Could you check a few things on this model? Use its own coordinates, in mm. A direction names the side the tool comes from. Round coordinates to 2 decimals unless told otherwise and drop trailing zeros. Write each loop counter-clockwise with the first axis right and the second up, starting at its lowest first coordinate (ties: lowest second). Pieces come first, ordered by that corner, then holes. Notation, with made-up numbers: (51, -3) -> (79, -3) arc R23 ccw to (79, 18) -> close; hole circle Ø2 at (73, -39.5). An arc over 180 degrees is marked (long way). Answer as CSV lines item,"result". Start each with the question number.
Q1. Imagine slicing it at A-A on y = 108. Please give me the cut outline in (x, z).
Q2. If we mould it in two halves opening along X, with no side actions, what happens to faces 6 (the cylindrical face through (54.55, 63.2, 0.93)), 7 (the cylindrical face through (-53.253, 56.857, 3.226)), 8 (the flat face through (-49.5, 73, 7)), 9 (the flat face through (-1, 115, 2))? For each: pulls with the +X half, pulls with the -X half, needs draft (parallel to the pull), parting line crosses it, or undercut.
Q3. Imagine slicing it at D-D on y = 62. Please give me the cut outline in (x, z), and give its area (3 significant figures).
Q4. Imagine slicing it at B-B on x = 0. Please give me the cut outline in (y, z).
Q5. Imagine slicing it at C-C on z = 6.25. Please give me the cut outline in (x, y), and give its area (3 significant figures).
Q6. Will these pins go through, and if not, where does the flat tip stop? pin 1 Ø4 at (x, y) = (59, 55.5) entering from -Z; pin 2 Ø10.5 at (x, y) = (0, 108) entering from +Z; pin 3 Ø2.5 at (x, z) = (-7, 3.5) entering from -Y; pin 4 Ø6 at (x, y) = (-50, 108) entering from +Z.
Q7. For faces 1 (the flat face through (-63.5, 81, 2)), 2 (the flat face through (-35.5, 73, 5)), 3 (the flat face through (59, 60, 1.5)), 4 (the flat face through (42, 74, 10)), 5 (the flat face through (-43, 100, 7)), which set-ups out of +Z, -Z, +X, -X, +Y, -Y let a thin tool reach every point of the face, with its end or its side?
Q8. If I drill on line 1 (X direction, y = 57, z = 0.45); line 2 (Y direction, x = 50, z = 2.5); line 3 (Y direction, x = 0, z = 1.9), over which ranges is the centre line in solid material (lowest first)? Write a range as [from, to].
from build123d import *

# Parameters (mm, degrees)
SKETCH2_R            = 3.25
BOSS_EXTRUDE2_DEPTH  = 5
SKETCH4_W            = 14
SKETCH4_H            = 53
RIBS_DEPTH           = 5
ANGLE_CUT_DEPTH      = 132.746916472
ANGLE_CUT_DEPTH_BACK = 132.746916472
SKETCH3_R            = 6.5
COUNTERBORE_DEPTH    = 1.5
SKETCH6_R            = 3.25
BOLT_THRU_HOLE_DEPTH = 105.895123001


with BuildPart() as part:
    # Sketch2 → Boss-Extrude2 (new body)
    with BuildSketch(Plane.XY):
        Polygon((-63.5, 47), (-63.5, 115), (63.5, 115), (63.5, 47), (35.5, 47), (35.5, 100), (-35.5, 100), (-35.5, 47), align=None)
        with Locations((-50, 108)):
            Circle(SKETCH2_R, mode=Mode.SUBTRACT)
        with Locations((50, 108)):
            Circle(SKETCH2_R, mode=Mode.SUBTRACT)
        with Locations((0, 108)):
            Circle(SKETCH2_R, mode=Mode.SUBTRACT)
    extrude(amount=BOSS_EXTRUDE2_DEPTH)

    # Sketch4 → Ribs (add)
    with BuildSketch(Plane.XY.offset(5)):
        with Locations((-42.5, 73.5)):
            Rectangle(SKETCH4_W, SKETCH4_H)
        with Locations((42.5, 73.5)):
            Rectangle(SKETCH4_W, SKETCH4_H)
    extrude(amount=RIBS_DEPTH)

    # Sketch5 → Angle Cut (cut, two sides: drawn at the far end of the back side and taken through both)
    with BuildSketch(Plane(origin=(0, 0, 0), x_dir=(0, 0, -1), z_dir=(1, 0, 0)).offset(-ANGLE_CUT_DEPTH_BACK)):
        Polygon((0, 47), (0, 65), (-0.628573851, 47), align=None)
    extrude(amount=ANGLE_CUT_DEPTH + ANGLE_CUT_DEPTH_BACK, mode=Mode.SUBTRACT)

    # Sketch3 → Counterbore (cut)
    with BuildSketch(Plane(origin=(0, 93.494633495, 0), x_dir=(-1, 0, 0), z_dir=(0, 0, 1))):
        with Locations(Location((56.5, 36.494633495, 0), (0, 0, 270))):
            Circle(SKETCH3_R)
        with Locations(Location((-56.5, 36.494633495, 0), (0, 0, 270))):
            Circle(SKETCH3_R)
    extrude(amount=COUNTERBORE_DEPTH, mode=Mode.SUBTRACT)

    # Sketch6 → Bolt thru-hole (cut, through all)
    with BuildSketch(Plane(origin=(0, 129.889907886, 0), x_dir=(-1, 0, 0), z_dir=(0, 0, 1))):
        with Locations((-56.5, 72.889907886)):
            Circle(SKETCH6_R)
        with Locations((56.5, 72.889907886)):
            Circle(SKETCH6_R)
    extrude(amount=BOLT_THRU_HOLE_DEPTH, mode=Mode.SUBTRACT)


solid = part.part
Checks:
1,outline,"(-63.5, 0) -> (-53.25, 0) -> (-53.25, 5) -> (-63.5, 5) -> close; (-46.75, 0) -> (-3.25, 0) -> (-3.25, 5) -> (-46.75, 5) -> close; (3.25, 0) -> (46.75, 0) -> (46.75, 5) -> (3.25, 5) -> close; (53.25, 0) -> (63.5, 0) -> (63.5, 5) -> (53.25, 5) -> close"
2,face 6,"undercut"
2,face 7,"undercut"
2,face 8,"pulls with the -X half"
2,face 9,"needs draft"
3,outline,"(-63.5, 0.1) -> (-60.65, 0.1) -> (-60.65, 1.5) -> (-52.35, 1.5) -> (-52.35, 0.1) -> (-35.5, 0.1) -> (-35.5, 10) -> (-49.5, 10) -> (-49.5, 5) -> (-63.5, 5) -> close; (35.5, 0.1) -> (52.35, 0.1) -> (52.35, 1.5) -> (60.65, 1.5) -> (60.65, 0.1) -> (63.5, 0.1) -> (63.5, 5) -> (49.5, 5) -> (49.5, 10) -> (35.5, 10) -> close"
3,area,"391 mm^2"
4,outline,"(100, 0) -> (104.75, 0) -> (104.75, 5) -> (100, 5) -> close; (111.25, 0) -> (115, 0) -> (115, 5) -> (111.25, 5) -> close"
5,outline,"(-49.5, 47) -> (-35.5, 47) -> (-35.5, 100) -> (-49.5, 100) -> close; (35.5, 47) -> (49.5, 47) -> (49.5, 100) -> (35.5, 100) -> close"
5,area,"1,480 mm^2"
6,pin 1,"z = 1.5"
6,pin 2,"z = 5"
6,pin 3,"y = 100"
6,pin 4,"through"
7,face 1,"+Z, -Z, -X, +Y, -Y"
7,face 2,"+Z, -Z, -Y"
7,face 3,"-Z"
7,face 4,"+Z, +X, -X, +Y, -Y"
7,face 5,"+Z, +X, -X, +Y"
8,line 1,"[-63.5, -63], [-50, -35.5], [35.5, 50], [63, 63.5]"
8,line 2,"[47, 104.75], [111.25, 115]"
8,line 3,"[100, 104.75], [111.25, 115]"
